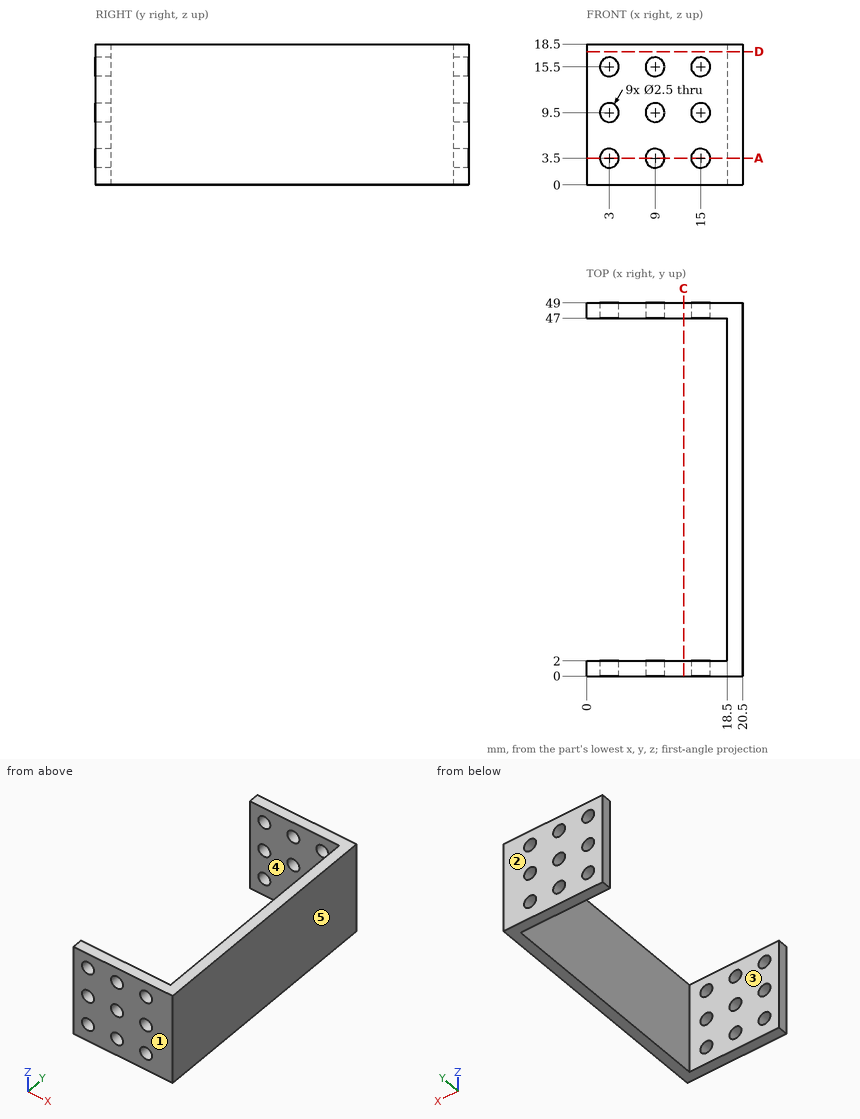
The figure shows three views and two pictorial views of one solid part (mm, origin at its lowest corner). Answer the questions. A direction names the side the tool comes from. Round coordinates to 2 decimals unless told otherwise and drop trailing zeros. Order: outer loops, then holes, each group sorted by start corner. A loop starts at its lowest first (then second) coordinate and runs counter-clockwise, first axis right, second up. Notation, with made-up numbers: M 71,13.5 L 77,13.5 A15 cw 77,42.5 Z; hole C 73,89.5 d1. An arc over 180 degrees is marked long. Answer in a Markdown table with one row per item. Add a question column.
1) The part is cut by section A-A on z = 3.5. Count the separate pieces of the cut face and the enclosed holes in it, plus the area to 3 significant figures.
2) Determine the mould class of the marked faces 1, 2 and 3 for opening direction Y: pulls with the +Y half, pulls with the -Y half, needs draft (parallel to the pull), parting line crosses it, or undercut.
3) Which of the six approach directions +Z, -Z, +X, -X, +Y, -Y give full straight-line access (tool end or side, diameter ignored) to the marked faces 4 and 5?
4) Flat-ended cylindrical pins translate along their axes: pin 1 Ø2 at (x, z) = (9, 15.5) entering from -Y; pin 2 Ø10 at (y, z) = (29, 3.5) entering from -X. Find the tip coordinate at first contact, or state that the pin passes through.
5) The part is cut by section D-D on z = 17.5. Determine the outline of the cut face in (x, y), plus the area to 3 significant figures.
6) The part is cut by section C-C on x = 12.75. Determine the outline of the cut face in (y, z).
7) Consider line 1 along Z through (x, y) = (3, 47.5); line 2 along Y through (x, z) = (6.75, 5.5); line 3 along X through (y, z) = (8, 3.5). Determine where each line is inside the solid, lowest interval first. Write a range as from..to.
Findings below:
| question | item | result |
|---|---|---|
| 1 | separate pieces | 7 |
| 1 | enclosed holes | 0 |
| 1 | area | 142 mm² |
| 2 | face 1 | pulls with the -Y half |
| 2 | face 2 | pulls with the +Y half |
| 2 | face 3 | undercut |
| 3 | face 4 | +Z, -Z, -X |
| 3 | face 5 | +Z, -Z, +X, +Y, -Y |
| 4 | pin 1 | passes through |
| 4 | pin 2 | stops at x = 18.5 |
| 5 | outline | M 0,0 L 20.5,0 L 20.5,49 L 0,49 L 0,47 L 18.5,47 L 18.5,2 L 0,2 Z |
| 5 | area | 172 mm² |
| 6 | outline | M 0,0 L 2,0 L 2,18.5 L 0,18.5 Z; M 47,0 L 49,0 L 49,18.5 L 47,18.5 Z |
| 7 | line 1 | z = 0..2.25, 4.75..8.25, 10.75..14.25, 16.75..18.5 |
| 7 | line 2 | y = 0..2, 47..49 |
| 7 | line 3 | x = 18.5..20.5 |
